```python
from build123d import *

# Parameters (mm, degrees)
SKETCH_1_W          = 7
SKETCH_1_H          = 4
EXTRUDE_1_DEPTH     = 4
CUT_EXTRUDE_1_DEPTH = 4
CUT_EXTRUDE_2_DEPTH = 6.4
CUT_EXTRUDE_3_DEPTH = 2
CUT_EXTRUDE_4_DEPTH = 3.8


with BuildPart() as part:
    # 草圖1 → 填料-伸長1 (new body)
    with BuildSketch(Plane(origin=(0, 0, 0), x_dir=(1, 0, 0), z_dir=(0, 1, 0))):
        Rectangle(SKETCH_1_W, SKETCH_1_H)
    extrude(amount=EXTRUDE_1_DEPTH)

    # 草圖2 → 除料-伸長1 (cut)
    with BuildSketch(Plane.XY.offset(2)):
        Polygon((3.5, 4), (-0.5, 4), (3.5, 2), align=None)
    extrude(amount=-CUT_EXTRUDE_1_DEPTH, mode=Mode.SUBTRACT)

    # 草圖3 → 除料-伸長2 (cut)
    with BuildSketch(Plane(origin=(0, 0, 0), x_dir=(1, 0, 0), z_dir=(0, 1, 0))):
        Polygon((-0.5, -2), (3.5, -2), (3.5, 0), align=None)
    extrude(amount=CUT_EXTRUDE_2_DEPTH, mode=Mode.SUBTRACT)

    # 草圖4 → 除料-伸長3 (cut)
    with BuildSketch(Plane(origin=(0, 4, 0), x_dir=(1, 0, 0), z_dir=(0, 1, 0))):
        Polygon((3.5, 0), (-0.5, 0), (-0.5, -2), align=None)
    extrude(amount=-CUT_EXTRUDE_3_DEPTH, mode=Mode.SUBTRACT)

    # 草圖5 → 除料-伸長4 (cut)
    with BuildSketch(Plane(origin=(-0.5, 0, 0), x_dir=(0, 0, -1), z_dir=(1, 0, 0))):
        Polygon((0, 4), (-2, 4), (-2, 2), align=None)
    extrude(amount=-CUT_EXTRUDE_4_DEPTH, mode=Mode.SUBTRACT)


solid = part.part
```
Can you work these out from the model? Positions are in its coordinate system, mm. A direction names the side the tool comes from. Give positions to 0.01 mm unless a question says otherwise; leave off trailing zeros. Order: outer loops, then holes, each group sorted by start corner. A loop starts at its lowest first (then second) coordinate and runs counter-clockwise, first axis right, second up. Notation, with made-up numbers: M 5.25,73 L 14.25,73 A23 ccw 14.25,100 Z; hole C 5.5,-33.5 d7. An arc over 180 degrees is marked long. One line per item, written item: value.
1) I want a section at B-B, the plane z = -1.4. List the corners of the cut face in (x, y) for me, plus the area to 3 significant figures.
Answer sheet:
outline: M -3.5,0 L 3.5,0 L 3.5,2 L -0.5,4 L -3.5,4 Z
area: 24.0 mm^2
2) For P1, Ø1, axis at y = 2, z = 1.5, coming from the +X side; P2, Ø2, axis at x = 1, z = 1.5, coming from the +Y side, each with a flat end and sliding along its axis, tell me the tip position at first contact or that it passes through.
Answer sheet:
P1: stops at x = 1.5
P2: stops at y = 2
3) On a 3-axis mill with a long thin cutter (end or side, diameter ignored), from which of +Z, -Z, +X, -X, +Y, -Y can I reach the whole of each face in a straight line? I mean faces 1 (the face through (1, 3, 0)), 2 (the face through (0, 0, 0)). Say none if no direction works.
Answer sheet:
face 1: +Z, +X, +Y
face 2: +Z, -Z, +X, -X, -Y
4) I want a section at C-C, the plane x = 0.5. List the corners of the cut face in (y, z) for me, plus the area to 3 significant figures.
Answer sheet:
outline: M 0,-2 L 3.5,-2 L 3.5,0 L 2,0 L 2,1.5 L 0,1.5 Z
area: 10.0 mm^2
5) I want a section at D-D, the plane y = 2.75. List the corners of the cut face in (x, z) for me, plus the area to 4 significant figures.
Answer sheet:
outline: M -3.5,-2 L 2,-2 L 2,0 L -0.5,0 L -0.5,1.25 L -3.5,1.25 Z
area: 14.75 mm^2
6) I want a section at A-A, the plane y = 1.2. List the corners of the cut face in (x, z) for me.
Answer sheet:
outline: M -3.5,-2 L 3.5,-2 L 3.5,0 L -0.5,2 L -3.5,2 Z
7) Please list where these lines run through material, in increasing order: line 1 along Y through (x, z) = (1.25, 0.5); line 2 along Z through (x, y) = (1.25, 2.8); line 3 along X through (y, z) = (2.2, 0.3).
Answer sheet:
line 1: y = 0 to 2
line 2: z = -2 to 0
line 3: x = -3.5 to -0.5
